```python
from build123d import *

# Parameters (mm, degrees)
SKETCH1_W                                         = 36
SKETCH1_H                                         = 9
BOSS_EXTRUDE1_DEPTH                               = 28
CUT_EXTRUDE1_DEPTH                                = 28
CUT_EXTRUDE2_DEPTH                                = 36
SKETCH5_W                                         = 11.440376565
SKETCH5_H                                         = 15.618965423
CUT_EXTRUDE4_DEPTH                                = 2
CUT_EXTRUDE5_DEPTH                                = 2
CUT_EXTRUDE5_DEPTH_BACK                           = 2
CUT_EXTRUDE6_DEPTH                                = 26
CUT_EXTRUDE7_DEPTH                                = 26
SKETCH10_R                                        = 3
CUT_EXTRUDE8_DEPTH                                = 7
SKETCH11_R                                        = 1.5
CUT_EXTRUDE9_DEPTH                                = 2
SKETCH12_R                                        = 1.5
CUT_EXTRUDE10_DEPTH                               = 9
CSK_FOR_3_FLAT_HEAD_MACHINE_SCREW_100_D           = 3.048
CSK_FOR_3_FLAT_HEAD_MACHINE_SCREW_100_DEPTH       = 9
CSK_FOR_3_FLAT_HEAD_MACHINE_SCREW_100_CSINK_D     = 5.0546
CSK_FOR_3_FLAT_HEAD_MACHINE_SCREW_100_CSINK_ANGLE = 100
SKETCH15_W                                        = 5.3
SKETCH15_H                                        = 5.3
CUT_EXTRUDE11_DEPTH                               = 2.5


with BuildPart() as part:
    # Sketch1 → Boss-Extrude1 (new body)
    with BuildSketch(Plane.XY):
        with Locations((18, 4.5)):
            Rectangle(SKETCH1_W, SKETCH1_H)
    extrude(amount=BOSS_EXTRUDE1_DEPTH)

    # Sketch2 → Cut-Extrude1 (cut)
    with BuildSketch(Plane.XY):
        Polygon((0, 4.5), (4.5, 9), (0, 9), align=None)
        Polygon((36, 4.5), (31.5, 9), (36, 9), align=None)
    extrude(amount=CUT_EXTRUDE1_DEPTH, mode=Mode.SUBTRACT)

    # Sketch3 → Cut-Extrude2 (cut)
    with BuildSketch(Plane(origin=(0, 0, 0), x_dir=(0, 0, -1), z_dir=(1, 0, 0))):
        Polygon((-28, 4.5), (-23.5, 9), (-28, 9), align=None)
    extrude(amount=CUT_EXTRUDE2_DEPTH, mode=Mode.SUBTRACT)

    # Sketch5 → Cut-Extrude4 (cut)
    with BuildSketch(Plane(origin=(32, 0, 32), x_dir=(0, 1, 0), z_dir=(0.707106781, 0, 0.707106781))):
        with Locations((5.720188283, -5.935696583)):
            Rectangle(SKETCH5_W, SKETCH5_H)
    extrude(amount=-CUT_EXTRUDE4_DEPTH, mode=Mode.SUBTRACT)

    # Sketch6 → Cut-Extrude5 (cut, two sides)
    with BuildSketch(Plane(origin=(4, 0, -4), x_dir=(0.577350269, -0.577350269, 0.577350269), z_dir=(-0.707106781, 0, 0.707106781))) as cut_extrude5_sk:
        Polygon((26.558112383, 29.802125204), (32.719347855, 28.647424665), (30.19862658, 32.212262879), align=None)
    extrude(amount=CUT_EXTRUDE5_DEPTH, mode=Mode.SUBTRACT)
    extrude(cut_extrude5_sk.sketch, amount=-CUT_EXTRUDE5_DEPTH_BACK, mode=Mode.SUBTRACT)

    # Sketch7 → Cut-Extrude6 (cut)
    with BuildSketch(Plane.XY):
        Polygon((5, 0), (5, 3), (5.707106781, 3.707106781), (13.104524105, 3.707106781), (13.811630886, 3), (13.811630886, 0), align=None)
    extrude(amount=CUT_EXTRUDE6_DEPTH, mode=Mode.SUBTRACT)

    # Sketch8 → Cut-Extrude7 (cut)
    with BuildSketch(Plane.XY.offset(28)):
        Polygon((36, 0), (30, 0), (34.5, 4.5), (34.5, 6), (36, 6), align=None)
    extrude(amount=-CUT_EXTRUDE7_DEPTH, mode=Mode.SUBTRACT)

    # Sketch10 → Cut-Extrude8 (cut)
    with BuildSketch(Plane(origin=(0, 9, 0), x_dir=(1, 0, 0), z_dir=(0, 1, 0))):
        with Locations((22, -6.5)):
            Circle(SKETCH10_R)
    extrude(amount=-CUT_EXTRUDE8_DEPTH, mode=Mode.SUBTRACT)

    # Sketch11 → Cut-Extrude9 (cut)
    with BuildSketch(Plane(origin=(0, 2, 0), x_dir=(1, 0, 0), z_dir=(0, 1, 0))):
        with Locations((22, -6.5)):
            Circle(SKETCH11_R)
    extrude(amount=-CUT_EXTRUDE9_DEPTH, mode=Mode.SUBTRACT)

    # Sketch12 → Cut-Extrude10 (cut)
    with BuildSketch(Plane(origin=(0, 0, 0), x_dir=(1, 0, 0), z_dir=(0, 1, 0))):
        with Locations((22, -16.5)):
            Circle(SKETCH12_R)
    extrude(amount=CUT_EXTRUDE10_DEPTH, mode=Mode.SUBTRACT)

    # CSK for #3 Flat Head Machine Screw (100)1
    with Locations(Plane(origin=(22, 9, 16.5), x_dir=(0, 0, 1), z_dir=(0, 1, 0))):
        with Locations((0, 0)):
            CounterSinkHole(CSK_FOR_3_FLAT_HEAD_MACHINE_SCREW_100_D / 2, CSK_FOR_3_FLAT_HEAD_MACHINE_SCREW_100_CSINK_D / 2, depth=CSK_FOR_3_FLAT_HEAD_MACHINE_SCREW_100_DEPTH, counter_sink_angle=CSK_FOR_3_FLAT_HEAD_MACHINE_SCREW_100_CSINK_ANGLE)

    # Sketch15 → Cut-Extrude11 (cut)
    with BuildSketch(Plane(origin=(0, 4.75, 0), x_dir=(1, 0, 0), z_dir=(0, 1, 0))):
        with Locations((22, -16.5)):
            Rectangle(SKETCH15_W, SKETCH15_H)
    extrude(amount=CUT_EXTRUDE11_DEPTH, mode=Mode.SUBTRACT)


solid = part.part
```
The model under review builds one solid part; all positions refer to its coordinate system, in mm. A direction names the side the tool comes from. Round coordinates to 2 decimals unless told otherwise and drop trailing zeros. Write each loop counter-clockwise with the first axis right and the second up, starting at its lowest first coordinate (ties: lowest second). Pieces come first, ordered by that corner, then holes.
(1) We need section B-B on z = 6.5. Give the boundary of the cut face in (x, y), and give its area (3 significant figures).
(2) Wall thickness on L1, parallel to X at y = 0.9, z = 6.5; L2, parallel to X at y = 3.35, z = 16.5; L3, parallel to Z at x = 22, y = 7: over which ranges is each line inside the solid? List them lowest first.
(3) Mouldability with a two-part tool opening along X and no side actions: class faces 5 (the flat face through (18, 9, 12)), 6 (the flat face through (34.5, 5, 15)), 7 (the flat face through (23, 7.25, 18)) as +X half, -X half, draft (parallel to the pull), parting line (faces both ways), or undercut.
(4) We need section A-A on x = 22. Give the boundary of the cut face in (y, z).
(5) We need section D-D on x = 9. Give the boundary of the cut face in (y, z), and give its area (3 significant figures).
(6) Insertion check: pin 1 (1.5 mm diameter, centred on y = 2.5, z = 7, fed in from +X); pin 2 (1.8 mm diameter, centred on x = 22, z = 6.5, fed in from -Y); pin 3 (0.8 mm diameter, centred on y = 5.5, z = 16.5, fed in from +X); pin 4 (3 mm diameter, centred on x = 8, y = 2, fed in from -Z). Each pin has a flat end and moves straight along its axis. Give the tip position at first contact, or say it passes through.
(7) Machinability: for faces 1 (the flat face through (22, 6, 13.85)), 2 (the flat face through (34, 2, 2)), 3 (the flat face through (13.812, 2, 13)), 4 (the flat face through (23, 2, 5)), which of the approach directions +Z, -Z, +X, -X, +Y, -Y give a long, thin tool a straight path to every point of the face, cutting with its end or side? Answer none if there is none.
(8) We need section C-C on y = 1.5. Give the boundary of the cut face in (x, z).
Findings below:
1. outline: (0, 0) - (5, 0) - (5, 3) - (5.71, 3.71) - (13.1, 3.71) - (13.81, 3) - (13.81, 0) - (20.5, 0) - (20.5, 2) - (19, 2) - (19, 9) - (4.5, 9) - (0, 4.5) - close; (23.5, 0) - (30, 0) - (34.5, 4.5) - (34.5, 6) - (31.5, 9) - (25, 9) - (25, 2) - (23.5, 2) - close
1. area: 206 mm2
2. L1: x = 0 to 5, 13.81 to 20.5, 23.5 to 30.9
2. L2: x = 0 to 5.35, 13.46 to 20.48, 23.52 to 33.35
2. L3: z = 0 to 3.5, 9.5 to 13.85, 19.15 to 25.5
3. face 5: draft
3. face 6: +X half
3. face 7: undercut
4. outline: (0, 0) - (9, 0) - (9, 3.5) - (2, 3.5) - (2, 5) - (0, 5) - close; (0, 8) - (2, 8) - (2, 9.5) - (9, 9.5) - (9, 13.97) - (8.16, 14.98) - (7.25, 14.98) - (7.25, 13.85) - (4.75, 13.85) - (4.75, 14.98) - (0, 14.98) - close; (0, 18.02) - (4.75, 18.02) - (4.75, 19.15) - (7.25, 19.15) - (7.25, 18.02) - (8.16, 18.02) - (9, 19.03) - (9, 23.5) - (4.5, 28) - (0, 28) - close
5. outline: (0, 26) - (3.71, 26) - (3.71, 0) - (9, 0) - (9, 23.5) - (4.5, 28) - (0, 28) - close
5. area: 145 mm2
6. pin 1: stops at x = 33.25
6. pin 2: passes through
6. pin 3: stops at x = 34.5
6. pin 4: stops at z = 26
7. face 1: none
7. face 2: +Z, +X, -Y
7. face 3: -Z, -Y
7. face 4: +Y
8. outline: (0, 0) - (5, 0) - (5, 26) - (13.81, 26) - (13.81, 0) - (36, 0) - (36, 2) - (31.5, 2) - (31.5, 28) - (0, 28) - close; hole circle Ø3.05 at (22, 16.5); hole circle Ø3 at (22, 6.5)
